The model under review builds one solid part; all positions refer to its coordinate system, in mm. A direction names the side the tool comes from. Round coordinates to 2 decimals unless told otherwise and drop trailing zeros. Loops run counter-clockwise (first coordinate to the right, second up) from the corner with the lowest first, then second, coordinate; pieces in that order, holes last. Notation, with made-up numbers: (35.25, 33.5) -> (71.25, 33.5) arc R25 cw to (71.25, 59.5) -> close; hole circle Ø10 at (24, 32.25). An arc over 180 degrees is marked (long way). Use a Markdown table: item, result. Add a question column.
1) Consider section B-B on x = 0. Give the boundary of the cut face in (y, z), plus the area to 3 significant figures.
2) Consider section C-C on z = 34.5. Give the boundary of the cut face in (x, y) (3 decimals), plus the area to 3 significant figures.
3) Consider section D-D on y = 0. State how many separate pieces and enclosed holes the cut face has, plus the area to 3 significant figures.
4) Mouldability with a two-part tool opening along Z and no side actions: class faces 1 (the cylindrical face through (35.361, -0.28, 2.755)), 2 (the flat face through (-7, -9, 45.5)), 3 (the flat face through (35, 0, 23)), 4 (the flat face through (-55.75, 0, 34)) as released by +Z, released by -Z, zero draft, split by the parting line, or undercut.
5) Insertion check: pin 1 (0.6 mm diameter, centred on y = -5, z = 7.5, fed in from +X); pin 2 (4.5 mm diameter, centred on x = -47, y = 4.5, fed in from -Z); pin 3 (4 mm diameter, centred on x = -49, y = 0, fed in from +Z) (3 decimals); pin 4 (18 mm diameter, centred on x = 0, y = 0, fed in from +Z). Each pin has a flat end and moves straight along its axis. Give the tip position at first contact, or say it passes through.
6) Consider section A-A on x = 28. Give the boundary of the cut face in (y, z).
7) Wall thickness on probe 1 along Y at (x, z) = (0, 43.65); probe 2 along Z at (x, y) = (-19, -11); probe 3 along X at (y, z) = (0, 43.6): over which ranges is each line inside the solid? List them lowest first.
8) For faces 5 (the flat face through (7, -9, 0.5)), 6 (the cylindrical face through (-34.14, -0.28, 3.9)), 7 (the flat face through (-42.8, -12.7, 35.8)), list the 3-axis set-ups (+Z, -Z, +X, -X, +Y, -Y) from which the entire face can be reached by the end or side of a thin tool; tool diameter is ignored.
from build123d import *

# Parameters (mm, degrees)
BOSS_EXTRUDE1_DEPTH                 = 20
BOSS_EXTRUDE1_DEPTH_BACK            = 20
FILLET1_R                           = 10
CUT_EXTRUDE1_DEPTH                  = 75.688101624
CUT_EXTRUDE1_DEPTH_BACK             = 75.688101624
CUT_EXTRUDE2_DEPTH                  = 10.375
CUT_EXTRUDE2_DIRECTION_2_REACH      = 76.688
CUT_EXTRUDE2_DIRECTION_2_END_RADIUS = 10
FILLET2_R                           = 10
FILLET3_R                           = 5
CUT_EXTRUDE3_DEPTH                  = 20
CUT_EXTRUDE4_DEPTH                  = 75.384558372
CUT_EXTRUDE4_DEPTH_BACK             = 75.384558372
SKETCH4_R                           = 10


with BuildPart() as part:
    # Sketch1 → Boss-Extrude1 (new, two sides: drawn at the far end of the back side and taken through both)
    with BuildSketch(Plane(origin=(0, 0, 0), x_dir=(1, 0, 0), z_dir=(0, 1, 0)).offset(-BOSS_EXTRUDE1_DEPTH_BACK)):
        with BuildLine():
            Line((-35, -33.125), (-55.75, -33.125))
            Line((-55.75, -33.125), (-55.75, -35.625))
            Line((-55.75, -35.625), (-37.5, -35.625))
            Line((-37.5, -35.625), (-37.5, -38))
            ThreePointArc((-37.5, -38), (-35.303300859, -43.303300859), (-30, -45.5))
            Line((-30, -45.5), (30, -45.5))
            ThreePointArc((30, -45.5), (35.303300859, -43.303300859), (37.5, -38))
            Line((37.5, -38), (37.5, -8))
            ThreePointArc((37.5, -8), (35.303300859, -2.696699141), (30, -0.5))
            Line((30, -0.5), (-30, -0.5))
            ThreePointArc((-30, -0.5), (-35.303300859, -2.696699141), (-37.5, -8))
            Line((-37.5, -8), (-37.5, -10.375))
            Line((-37.5, -10.375), (-55.75, -10.375))
            Line((-55.75, -10.375), (-55.75, -12.875))
            Line((-55.75, -12.875), (-35, -12.875))
            Line((-35, -12.875), (-35, -6))
            ThreePointArc((-35, -6), (-34.121320344, -3.878679656), (-32, -3))
            Line((-32, -3), (32, -3))
            ThreePointArc((32, -3), (34.121320344, -3.878679656), (35, -6))
            Line((35, -6), (35, -40))
            ThreePointArc((35, -40), (34.121320344, -42.121320344), (32, -43))
            Line((32, -43), (-32, -43))
            ThreePointArc((-32, -43), (-34.121320344, -42.121320344), (-35, -40))
            Line((-35, -40), (-35, -33.125))
        make_face()
    extrude(amount=BOSS_EXTRUDE1_DEPTH + BOSS_EXTRUDE1_DEPTH_BACK)

    # Fillet1
    fillet1_edges = [part.edges().sort_by_distance(p)[0] for p in [
        (-37.5, 0, 10.375),
        (-37.5, 0, 35.625),
    ]]
    fillet(fillet1_edges, radius=FILLET1_R)

    # Sketch2 → Cut-Extrude1 (cut, two sides: drawn at the far end of the back side and taken through both)
    with BuildSketch(Plane.XY.offset(-CUT_EXTRUDE1_DEPTH_BACK)):
        with BuildLine():
            ThreePointArc((-43.5, -10), (-44.12239809, -8.49739809), (-45.625, -7.875))
            Line((-45.625, -7.875), (-45.625, -12.125))
            ThreePointArc((-45.625, -12.125), (-44.12239809, -11.50260191), (-43.5, -10))
        make_face()
        with BuildLine():
            Line((-45.625, -12.125), (-45.625, -7.875))
            ThreePointArc((-45.625, -7.875), (-47.75, -10), (-45.625, -12.125))
        make_face()
        with BuildLine():
            ThreePointArc((-43.5, 10), (-44.12239809, 11.50260191), (-45.625, 12.125))
            Line((-45.625, 12.125), (-45.625, 7.875))
            ThreePointArc((-45.625, 7.875), (-44.12239809, 8.49739809), (-43.5, 10))
        make_face()
        with BuildLine():
            Line((-45.625, 7.875), (-45.625, 12.125))
            ThreePointArc((-45.625, 12.125), (-47.75, 10), (-45.625, 7.875))
        make_face()
    extrude(amount=CUT_EXTRUDE1_DEPTH + CUT_EXTRUDE1_DEPTH_BACK, mode=Mode.SUBTRACT)

    # Sketch2<4> → Cut-Extrude2 (cut)
    with BuildSketch(Plane.XY):
        with BuildLine():
            ThreePointArc((-41.375, 10), (-42.61979618, 13.00520382), (-45.625, 14.25))
            Line((-45.625, 14.25), (-45.625, 12.125))
            ThreePointArc((-45.625, 12.125), (-44.12239809, 11.50260191), (-43.5, 10))
            ThreePointArc((-43.5, 10), (-44.12239809, 8.49739809), (-45.625, 7.875))
            Line((-45.625, 7.875), (-45.625, 5.75))
            ThreePointArc((-45.625, 5.75), (-42.61979618, 6.99479618), (-41.375, 10))
        make_face()
        with BuildLine():
            Line((-45.625, 12.125), (-45.625, 14.25))
            ThreePointArc((-45.625, 14.25), (-49.875, 10), (-45.625, 5.75))
            Line((-45.625, 5.75), (-45.625, 7.875))
            ThreePointArc((-45.625, 7.875), (-47.75, 10), (-45.625, 12.125))
        make_face()
        with BuildLine():
            ThreePointArc((-41.375, -10), (-42.61979618, -6.99479618), (-45.625, -5.75))
            Line((-45.625, -5.75), (-45.625, -7.875))
            ThreePointArc((-45.625, -7.875), (-44.12239809, -8.49739809), (-43.5, -10))
            ThreePointArc((-43.5, -10), (-44.12239809, -11.50260191), (-45.625, -12.125))
            Line((-45.625, -12.125), (-45.625, -14.25))
            ThreePointArc((-45.625, -14.25), (-42.61979618, -13.00520382), (-41.375, -10))
        make_face()
        with BuildLine():
            Line((-45.625, -7.875), (-45.625, -5.75))
            ThreePointArc((-45.625, -5.75), (-49.875, -10), (-45.625, -14.25))
            Line((-45.625, -14.25), (-45.625, -12.125))
            ThreePointArc((-45.625, -12.125), (-47.75, -10), (-45.625, -7.875))
        make_face()
    extrude(amount=CUT_EXTRUDE2_DEPTH, mode=Mode.SUBTRACT)

    # Cut-Extrude2 direction 2: up to this cylinder (the profile starts inside it)
    cut_extrude2_direction_2_end = Plane(origin=(-45.751488025, -2.938005, 0.375), z_dir=(0, 1, 0)) * Cylinder(CUT_EXTRUDE2_DIRECTION_2_END_RADIUS, 194.376, mode=Mode.PRIVATE)
    # Sketch2<4> → Cut-Extrude2 direction 2 (cut, up to the surface)
    with BuildSketch(Plane.XY, mode=Mode.PRIVATE) as cut_extrude2_direction_2_sk1:
        with BuildLine():
            ThreePointArc((-41.375, 10), (-42.61979618, 13.00520382), (-45.625, 14.25))
            Line((-45.625, 14.25), (-45.625, 12.125))
            ThreePointArc((-45.625, 12.125), (-44.12239809, 11.50260191), (-43.5, 10))
            ThreePointArc((-43.5, 10), (-44.12239809, 8.49739809), (-45.625, 7.875))
            Line((-45.625, 7.875), (-45.625, 5.75))
            ThreePointArc((-45.625, 5.75), (-42.61979618, 6.99479618), (-41.375, 10))
        make_face()
    cut_extrude2_direction_2_tool1 = extrude(cut_extrude2_direction_2_sk1.sketch, amount=-CUT_EXTRUDE2_DIRECTION_2_REACH, mode=Mode.PRIVATE) & cut_extrude2_direction_2_end
    add(cut_extrude2_direction_2_tool1.solids().sort_by_distance((-42.686995, 7.061995, 0))[0], mode=Mode.SUBTRACT)
    # Sketch2<4> → Cut-Extrude2 direction 2 (cut, up to the surface)
    with BuildSketch(Plane.XY, mode=Mode.PRIVATE) as cut_extrude2_direction_2_sk2:
        with BuildLine():
            Line((-45.625, 12.125), (-45.625, 14.25))
            ThreePointArc((-45.625, 14.25), (-49.875, 10), (-45.625, 5.75))
            Line((-45.625, 5.75), (-45.625, 7.875))
            ThreePointArc((-45.625, 7.875), (-47.75, 10), (-45.625, 12.125))
        make_face()
    cut_extrude2_direction_2_tool2 = extrude(cut_extrude2_direction_2_sk2.sketch, amount=-CUT_EXTRUDE2_DIRECTION_2_REACH, mode=Mode.PRIVATE) & cut_extrude2_direction_2_end
    add(cut_extrude2_direction_2_tool2.solids().sort_by_distance((-45.720033, 6.8125, 0))[0], mode=Mode.SUBTRACT)
    # Sketch2<4> → Cut-Extrude2 direction 2 (cut, up to the surface)
    with BuildSketch(Plane.XY, mode=Mode.PRIVATE) as cut_extrude2_direction_2_sk3:
        with BuildLine():
            ThreePointArc((-41.375, -10), (-42.61979618, -6.99479618), (-45.625, -5.75))
            Line((-45.625, -5.75), (-45.625, -7.875))
            ThreePointArc((-45.625, -7.875), (-44.12239809, -8.49739809), (-43.5, -10))
            ThreePointArc((-43.5, -10), (-44.12239809, -11.50260191), (-45.625, -12.125))
            Line((-45.625, -12.125), (-45.625, -14.25))
            ThreePointArc((-45.625, -14.25), (-42.61979618, -13.00520382), (-41.375, -10))
        make_face()
    cut_extrude2_direction_2_tool3 = extrude(cut_extrude2_direction_2_sk3.sketch, amount=-CUT_EXTRUDE2_DIRECTION_2_REACH, mode=Mode.PRIVATE) & cut_extrude2_direction_2_end
    add(cut_extrude2_direction_2_tool3.solids().sort_by_distance((-42.686995, -12.938005, 0))[0], mode=Mode.SUBTRACT)
    # Sketch2<4> → Cut-Extrude2 direction 2 (cut, up to the surface)
    with BuildSketch(Plane.XY, mode=Mode.PRIVATE) as cut_extrude2_direction_2_sk4:
        with BuildLine():
            Line((-45.625, -7.875), (-45.625, -5.75))
            ThreePointArc((-45.625, -5.75), (-49.875, -10), (-45.625, -14.25))
            Line((-45.625, -14.25), (-45.625, -12.125))
            ThreePointArc((-45.625, -12.125), (-47.75, -10), (-45.625, -7.875))
        make_face()
    cut_extrude2_direction_2_tool4 = extrude(cut_extrude2_direction_2_sk4.sketch, amount=-CUT_EXTRUDE2_DIRECTION_2_REACH, mode=Mode.PRIVATE) & cut_extrude2_direction_2_end
    add(cut_extrude2_direction_2_tool4.solids().sort_by_distance((-49.779967, -10, 0))[0], mode=Mode.SUBTRACT)

    # Fillet2
    # the kernel refuses this fillet: 10 mm, written as the material it takes off along each edge
    with BuildSketch(Plane(origin=(-55.75, 20, -14.625), x_dir=(1, 0, 0), z_dir=(0, 0, 1)), Plane(origin=(-55.75, 20, 8.125), x_dir=(1, 0, 0), z_dir=(0, 0, 1))) as fillet2_piece_1:
        with BuildLine():
            CenterArc((FILLET2_R, -FILLET2_R), FILLET2_R, 90, 90)
            Line((0, -FILLET2_R), (0, 0))
            Line((0, 0), (FILLET2_R, 0))
        make_face()
    extrude(amount=52.5, mode=Mode.SUBTRACT)
    with BuildSketch(Plane(origin=(-55.75, -20, -14.625), x_dir=(1, 0, 0), z_dir=(0, 0, 1)), Plane(origin=(-55.75, -20, 8.125), x_dir=(1, 0, 0), z_dir=(0, 0, 1))) as fillet2_piece_2:
        with BuildLine():
            CenterArc((FILLET2_R, FILLET2_R), FILLET2_R, 180, 90)
            Line((0, FILLET2_R), (0, 0))
            Line((0, 0), (FILLET2_R, 0))
        make_face()
    extrude(amount=52.5, mode=Mode.SUBTRACT)

    # Fillet3
    fillet3_edges = [part.edges().sort_by_distance(p)[0] for p in [
        (-35, 0, 33.125),
        (-35, 0, 12.875),
    ]]
    fillet(fillet3_edges, radius=FILLET3_R)

    # Sketch3 → Cut-Extrude3 (cut)
    with BuildSketch(Plane.XY.offset(35.625)):
        Polygon((-45.625, 14.330127019), (-49.375, 12.165063509), (-49.375, 7.834936491), (-45.625, 5.669872981), (-41.875, 7.834936491), (-41.875, 12.165063509), align=None)
        Polygon((-45.625, -5.669872981), (-49.375, -7.834936491), (-49.375, -12.165063509), (-45.625, -14.330127019), (-41.875, -12.165063509), (-41.875, -7.834936491), align=None)
    extrude(amount=CUT_EXTRUDE3_DEPTH, mode=Mode.SUBTRACT)

    # Sketch4 → Cut-Extrude4 (cut, two sides: drawn at the far end of the back side and taken through both)
    with BuildSketch(Plane.XY.offset(45.5).offset(-CUT_EXTRUDE4_DEPTH_BACK)):
        Circle(SKETCH4_R)
    extrude(amount=CUT_EXTRUDE4_DEPTH + CUT_EXTRUDE4_DEPTH_BACK, mode=Mode.SUBTRACT)


solid = part.part
Result set:
| question | item | result |
|---|---|---|
| 1 | outline | (-20, 0.5) -> (-10, 0.5) -> (-10, 3) -> (-20, 3) -> close; (-20, 43) -> (-10, 43) -> (-10, 45.5) -> (-20, 45.5) -> close; (10, 0.5) -> (20, 0.5) -> (20, 3) -> (10, 3) -> close; (10, 43) -> (20, 43) -> (20, 45.5) -> (10, 45.5) -> close |
| 1 | area | 100 mm2 |
| 2 | outline | (-55.75, -10) arc R10 ccw to (-45.75, -20) -> (-36.556, -20) -> (-36.556, 20) -> (-45.75, 20) arc R10 ccw to (-55.75, 10) -> close; (35, -20) -> (37.5, -20) -> (37.5, 20) -> (35, 20) -> close; hole circle Ø4.25 at (-45.625, -10); hole circle Ø4.25 at (-45.625, 10) |
| 2 | area | 796 mm2 |
| 3 | separate pieces | 3 |
| 3 | enclosed holes | 0 |
| 3 | area | 486 mm2 |
| 4 | face 1 | released by -Z |
| 4 | face 2 | released by +Z |
| 4 | face 3 | undercut |
| 4 | face 4 | zero draft |
| 5 | pin 1 | x = 37.5 |
| 5 | pin 2 | z = 10.32 |
| 5 | pin 3 | z = 35.625 |
| 5 | pin 4 | through |
| 6 | outline | (-20, 0.5) -> (20, 0.5) -> (20, 3) -> (-20, 3) -> close; (-20, 43) -> (20, 43) -> (20, 45.5) -> (-20, 45.5) -> close |
| 7 | probe 1 | -20 to -10, 10 to 20 |
| 7 | probe 2 | 0.5 to 3, 43 to 45.5 |
| 7 | probe 3 | -34.99 to -10, 10 to 34.99 |
| 8 | face 5 | -Z, +X, -X, +Y, -Y |
| 8 | face 6 | +Y, -Y |
| 8 | face 7 | +Z, -X |
